Part model, mm, in its own coordinate system. Face numbers are marked on the shaded views. A direction names the side the tool comes from. Give positions to 0.01 mm unless a question says otherwise; leave off trailing zeros. Order: outer loops, then holes, each group sorted by start corner. A loop starts at its lowest first (then second) coordinate and runs counter-clockwise, first axis right, second up. Notation, with made-up numbers: M 88.25,35.25 L 110.25,35.25 A22 ccw 110.25,56.25 Z; hole C -36.75,-39.5 d7. An arc over 180 degrees is marked long. One line per question, with ' | ' between items.
```python
from build123d import *

# Parameters (mm, degrees)
F0_R     = 11.05
F0_R_2   = 5.524841
F0_R_3   = 5.521717
F1_DEPTH = 7


with BuildPart() as f1:
    # F0 (on Top) → F1 (new body)
    with BuildSketch(Plane.XY):
        with BuildLine():
            ThreePointArc((-30.27175, -3.219667), (-32.865041, -3.5851), (-35.339594, -4.442586))
            ThreePointArc((-35.339594, -4.442586), (-40.732584, -24.604776), (-19.918734, -26.148118))
            ThreePointArc((-19.918734, -26.148118), (-18.338716, -24.161725), (-17.156869, -21.915518))
            ThreePointArc((-17.156869, -21.915518), (-16.394062, -19.386242), (-16.136531, -16.757023))
            ThreePointArc((-16.136531, -16.757023), (-16.266635, -14.883817), (-16.65445, -13.046583))
            ThreePointArc((-16.65445, -13.046583), (-17.164663, -11.579637), (-17.839394, -10.180713))
            ThreePointArc((-17.839394, -10.180713), (-18.394537, -9.267472), (-19.019928, -8.400823))
            ThreePointArc((-19.019928, -8.400823), (-24.019109, -4.449187), (-30.27175, -3.219667))
        make_face()
        with Locations((-29.686531, -16.757023)):
            Circle(F0_R, mode=Mode.SUBTRACT)
        with BuildLine():
            ThreePointArc((-13.040381, 30.786681), (-12.067165, 28.448015), (-10.675671, 26.331354))
            ThreePointArc((-10.675671, 26.331354), (-6.029005, 22.482823), (-0.172342, 21.032925))
            ThreePointArc((-0.172342, 21.032925), (0.382199, 21.034199), (0.936224, 21.058163))
            ThreePointArc((0.936224, 21.058163), (6.867395, 22.856804), (11.377187, 27.108354))
            ThreePointArc((11.377187, 27.108354), (12.556434, 29.374864), (13.289258, 31.822448))
            ThreePointArc((13.289258, 31.822448), (-0.532624, 48.007374), (-13.040381, 30.786681))
        make_face()
        with Locations((0, 34.467846)):
            Circle(F0_R, mode=Mode.SUBTRACT)
        with BuildLine():
            ThreePointArc((0.952624, 20.951374), (0.388404, 20.923414), (-0.17649, 20.918996))
            ThreePointArc((-0.17649, 20.918996), (-9.648186, 15.43491), (-10.675671, 26.331354))
            ThreePointArc((-10.675671, 26.331354), (-12.067165, 28.448015), (-13.040381, 30.786681))
            ThreePointArc((-13.040381, 30.786681), (-17.005323, 26.255064), (-18.1368, 20.341006))
            ThreePointArc((-18.1368, 20.341006), (-27.800797, 16.327475), (-29.222287, 5.960189))
            ThreePointArc((-29.222287, 5.960189), (-33.762662, 1.630121), (-35.339594, -4.442586))
            ThreePointArc((-35.339594, -4.442586), (-32.865041, -3.5851), (-30.27175, -3.219667))
            ThreePointArc((-30.27175, -3.219667), (-21.194494, 1.684977), (-19.019928, -8.400823))
            ThreePointArc((-19.019928, -8.400823), (-18.394537, -9.267472), (-17.839394, -10.180713))
            ThreePointArc((-17.839394, -10.180713), (-8.23761, -15.509501), (-17.156869, -21.915518))
            ThreePointArc((-17.156869, -21.915518), (-18.338716, -24.161725), (-19.918734, -26.148118))
            ThreePointArc((-19.918734, -26.148118), (-14.644184, -27.386623), (-9.387936, -26.072605))
            ThreePointArc((-9.387936, -26.072605), (-1.069433, -31.784934), (8.232154, -27.872304))
            ThreePointArc((8.232154, -27.872304), (14.704134, -29.596756), (21.039259, -27.422716))
            ThreePointArc((21.039259, -27.422716), (19.240377, -25.683208), (17.792045, -23.642571))
            ThreePointArc((17.792045, -23.642571), (7.868212, -18.677143), (16.821859, -12.12198))
            ThreePointArc((16.821859, -12.12198), (17.329602, -10.93555), (17.947911, -9.802803))
            ThreePointArc((17.947911, -9.802803), (17.907438, 1.147655), (27.866747, -3.404964))
            ThreePointArc((27.866747, -3.404964), (30.35929, -3.329972), (32.823366, -3.71302))
            ThreePointArc((32.823366, -3.71302), (32.834455, -3.230002), (32.823366, -2.746983))
            ThreePointArc((32.823366, -2.746983), (30.747102, 2.4274), (26.48104, 6.017083))
            ThreePointArc((26.48104, 6.017083), (26.74913, 15.790636), (18.861073, 21.567552))
            ThreePointArc((18.861073, 21.567552), (17.472712, 27.454332), (13.289258, 31.822448))
            ThreePointArc((13.289258, 31.822448), (12.556434, 29.374864), (11.377187, 27.108354))
            ThreePointArc((11.377187, 27.108354), (10.674436, 16.394645), (0.952624, 20.951374))
        make_face()
        with Locations((0, -21.314567)):
            Circle(F0_R_2, mode=Mode.SUBTRACT)
        Circle(F0_R, mode=Mode.SUBTRACT)
        with Locations((-19.467567, 9.903785)):
            Circle(F0_R_3, mode=Mode.SUBTRACT)
        with BuildLine():
            ThreePointArc((-9.156847, 9.984555), (-9.053526, 10.078335), (-8.949245, 10.171047))
            ThreePointArc((-8.949245, 10.171047), (-8.946944, 10.055484), (-8.945912, 9.939903))
            ThreePointArc((-8.945912, 9.939903), (-9.051484, 9.961735), (-9.156847, 9.984555))
        make_face(mode=Mode.SUBTRACT)
        with Locations((17.297982, 11.159429)):
            Circle(F0_R_2, mode=Mode.SUBTRACT)
        with BuildLine():
            ThreePointArc((43.068773, -16.853878), (40.204739, -8.522454), (32.823366, -3.71302))
            ThreePointArc((32.823366, -3.71302), (30.35929, -3.329972), (27.866747, -3.404964))
            ThreePointArc((27.866747, -3.404964), (22.174096, -5.467122), (17.947911, -9.802803))
            ThreePointArc((17.947911, -9.802803), (17.329602, -10.93555), (16.821859, -12.12198))
            ThreePointArc((16.821859, -12.12198), (16.016566, -17.990943), (17.792045, -23.642571))
            ThreePointArc((17.792045, -23.642571), (19.240377, -25.683208), (21.039259, -27.422716))
            ThreePointArc((21.039259, -27.422716), (35.379877, -29.070669), (43.068773, -16.853878))
        make_face()
        with Locations((29.518773, -16.853878)):
            Circle(F0_R, mode=Mode.SUBTRACT)
    extrude(amount=F1_DEPTH)


solid = f1.part
```
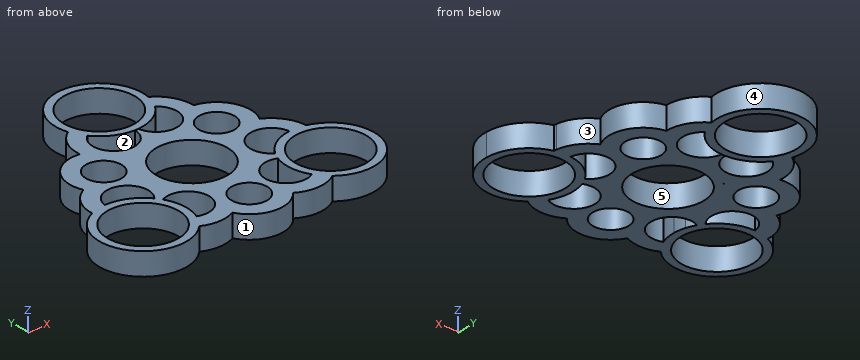
1. Drop flat-ended pins along their axis: pin 1 (1.5 mm diameter, centred on y = 23, z = 2.5, fed in from +X); pin 2 (6.5 mm diameter, centred on x = 17.3, y = 11.16, fed in from +Z); pin 3 (1 mm diameter, centred on y = 37, z = 3, fed in from -X); pin 4 (2 mm diameter, centred on y = -19, z = 3.5, fed in from -X). Give the stop position or say it passes through.
Worked out:
pin 1: stops at x = 18.86 | pin 2: passes through | pin 3: stops at x = -13.4 | pin 4: stops at x = -43.18
2. Mould opens along X. For the marked faces 3, 4 and 5 say: released by +X, released by -X, zero draft, split by the parting line, or undercut.
Worked out:
face 3: released by +X | face 4: split by the parting line | face 5: undercut
3. Slice it at D-D on y = 35.5. Give the cut face in (x, z).
Worked out:
outline: M -13.51,0 L -11,0 L -11,7 L -13.51,7 Z; M 11,0 L 13.51,0 L 13.51,7 L 11,7 Z
4. Slice it at C-C on x = 10. Give the cut face in (y, z), then the cut area to 3 significant figures.
Worked out:
outline: M -28.77,0 L -22.97,0 L -22.97,7 L -28.77,7 Z; M -13.3,0 L -4.7,0 L -4.7,7 L -13.3,7 Z; M 4.7,0 L 16.05,0 L 16.05,7 L 4.7,7 Z; M 25.36,0 L 29.77,0 L 29.77,7 L 25.36,7 Z; M 39.17,0 L 43.61,0 L 43.61,7 L 39.17,7 Z | area: 242 mm2
5. Slice it at B-B on y = 0. Give the cut face in (x, z).
Worked out:
outline: M -34.55,0 L -28.81,0 L -28.81,7 L -34.55,7 Z; M -18.97,0 L -11.05,0 L -11.05,7 L -18.97,7 Z; M 11.05,0 L 16.57,0 L 16.57,7 L 11.05,7 Z; M 26.29,0 L 32.09,0 L 32.09,7 L 26.29,7 Z
6. Slice it at A-A on x = -32. Give the cut face in (y, z), then the cut area to 3 significant figures.
Worked out:
outline: M -30.11,0 L -27.56,0 L -27.56,7 L -30.11,7 Z; M -5.95,0 L 3.91,0 L 3.91,7 L -5.95,7 Z | area: 86.9 mm2
7. Tool access for the marked faces 1 and 2: list every direction of +Z, -Z, +X, -X, +Y, -Y with a clear straight run to the whole face (end or side of a thin tool).
Worked out:
face 1: +Z, -Z, -Y | face 2: +Z, -Z
8. Probe L1, parallel to Y at x = -25.5, z = 3.25; L2, parallel to Y at x = -10, z = 2.5; L3, parallel to Y at x = -11.5, z = 2.25. List the from-to ranges inside material, lowest first. Write a range as from..to.
Worked out:
L1: y = -29.64..-26.98, -6.53..-3.87, 2.07..18.52 | L2: y = -26.37..-20.35, -11.42..-4.7, 4.7..15.63, 25.52..29.77, 39.17..43.61 | L3: y = -26.92..-21.53, -10.24..16.86, 25.56..41.63
